CAD build for the part. Positions are in the model's coordinates, mm. A direction names the side the tool comes from. Round coordinates to 2 decimals unless told otherwise and drop trailing zeros. Order: outer loops, then holes, each group sorted by start corner. A loop starts at its lowest first (then second) coordinate and runs counter-clockwise, first axis right, second up. Notation, with made-up numbers: M 80,16 L 116,16 A24 cw 116,43 Z; hole C -28.5,66.5 d11. An arc over 180 degrees is marked long. Answer as a JSON object with one key per item and string values. Group by question number.
```python
from build123d import *

# Parameters (mm, degrees)
BOSS_EXTRUDE1_DEPTH = 10
SKETCH2_R           = 1.75
CUT_EXTRUDE1_DEPTH  = 10
SKETCH3_R           = 21.1
CUT_EXTRUDE2_DEPTH  = 9
SKETCH4_R           = 7.5
CUT_EXTRUDE3_DEPTH  = 10


with BuildPart() as part:
    # Sketch1 → Boss-Extrude1 (new body)
    with BuildSketch(Plane.XY):
        with BuildLine():
            Line((-20.631764929, -8.976651708), (-20.631764929, -80.4))
            Line((-20.631764929, -80.4), (20.631764929, -80.4))
            Line((20.631764929, -80.4), (20.631764929, -8.976651708))
            ThreePointArc((20.631764929, -8.976651708), (0, 22.5), (-20.631764929, -8.976651708))
        make_face()
    extrude(amount=BOSS_EXTRUDE1_DEPTH)

    # Sketch2 → Cut-Extrude1 (cut)
    with BuildSketch(Plane(origin=(0, 0, 0), x_dir=(-1, 0, 0), z_dir=(0, 0, -1))):
        with Locations((0, 15)):
            Circle(SKETCH2_R)
        with Locations((12.990381057, -7.5)):
            Circle(SKETCH2_R)
        with Locations((-12.990381057, -7.5)):
            Circle(SKETCH2_R)
    extrude(amount=-CUT_EXTRUDE1_DEPTH, mode=Mode.SUBTRACT)

    # Sketch3 → Cut-Extrude2 (cut)
    with BuildSketch(Plane(origin=(0, 0, 0), x_dir=(-1, 0, 0), z_dir=(0, 0, -1))):
        Circle(SKETCH3_R)
    extrude(amount=-CUT_EXTRUDE2_DEPTH, mode=Mode.SUBTRACT)

    # Sketch4 → Cut-Extrude3 (cut)
    with BuildSketch(Plane(origin=(0, 0, 0), x_dir=(-1, 0, 0), z_dir=(0, 0, -1))):
        Circle(SKETCH4_R)
    extrude(amount=-CUT_EXTRUDE3_DEPTH, mode=Mode.SUBTRACT)


solid = part.part
```
Item 1: Cut at D-D, the plane x = -12.5. Give the cut face in (y, z), and give its area (3 significant figures).
Item 2: Cut at C-C, the plane z = 2. Give the cut face in (x, y).
Item 3: Cut at A-A, the plane y = 0. Give the cut face in (x, z), and give its area (3 significant figures).
Item 4: Drill centre lines: line 1 (Y direction, x = 0, z = 9.65); line 2 (Y direction, x = 0, z = 5); line 3 (Y direction, x = -10, z = 3.25). Where is each one in solid material? Low to high. Write a range as [from, to].
Item 5: Two-plate mould, pull along Y, no slides. Class faces 1 (the face through (0, -28, 10)), 2 (the face through (0.62, 22.49, 4.93)), 3 (the face through (-20.126, 6.338, 4.437)): +Y half, -Y half, draft (parallel to the pull), parting line (faces both ways), or undercut.
Item 6: 3-axis set-ups, long thin cutter, end or side, ignore diameter. For faces 4 (the face through (-20.632, -44, 5)), 5 (the face through (0, -51, 0)), 6 (the face through (-14.607, -8.17, 9.493)), 7 (the face through (20.632, -45, 5)), 8 (the face through (0, -9, 9)): which of +Z, -Z, +X, -X, +Y, -Y reach the whole face in a straight line?
Item 7: Flat gauge pins, fed straight in: pin 1 Ø3 at (x, y) = (-12.99, -7.5) entering from -Z; pin 2 Ø3 at (y, z) = (-13, 6) entering from -X; pin 3 Ø4 at (x, y) = (12.99, -7.5) entering from -Z; pin 4 Ø1 at (x, z) = (0.5, 7) entering from +Y. Where does each tip first touch, or does it go through?
Item 8: Cut at B-B, the plane x = 0. Give the cut face in (y, z).
Response values:
{
 "1": {"outline": "M -80.4,0 L -17,0 L -17,9 L -9.18,9 L -9.18,10 L -80.4,10 Z; M -5.82,9 L 17,9 L 17,0 L 18.71,0 L 18.71,10 L -5.82,10 Z", "area": "682 mm^2"},
 "2": {"outline": "M -20.63,-80.4 L 20.63,-80.4 L 20.63,-8.98 A22.5 ccw long -20.63,-8.98 Z; hole C 0,0 d42.2"},
 "3": {"outline": "M -22.5,0 L -21.1,0 L -21.1,9 L -7.5,9 L -7.5,10 L -22.5,10 Z; M 7.5,9 L 21.1,9 L 21.1,0 L 22.5,0 L 22.5,10 L 7.5,10 Z", "area": "55.2 mm^2"},
 "4": {"line 1": "[-80.4, -7.5], [7.5, 13.25], [16.75, 22.5]", "line 2": "[-80.4, -21.1], [21.1, 22.5]", "line 3": "[-80.4, -18.58], [18.58, 20.16]"},
 "5": {"face 1": "draft", "face 2": "parting line", "face 3": "undercut"},
 "6": {"face 4": "+Z, -Z, -X, -Y", "face 5": "-Z, +X, -X, +Y, -Y", "face 6": "+Z, -Z", "face 7": "+Z, -Z, +X, -Y", "face 8": "-Z"},
 "7": {"pin 1": "through", "pin 2": "x = -20.63", "pin 3": "z = 9", "pin 4": "y = 22.5"},
 "8": {"outline": "M -80.4,0 L -21.1,0 L -21.1,9 L -7.5,9 L -7.5,10 L -80.4,10 Z; M 7.5,9 L 13.25,9 L 13.25,10 L 7.5,10 Z; M 16.75,9 L 21.1,9 L 21.1,0 L 22.5,0 L 22.5,10 L 16.75,10 Z"}
}
